Build history of the part. All positions in model axes, mm. A direction names the side the tool comes from. Round coordinates to 2 decimals unless told otherwise and drop trailing zeros. Write each loop counter-clockwise with the first axis right and the second up, starting at its lowest first coordinate (ties: lowest second). Pieces come first, ordered by that corner, then holes.
from build123d import *

# Parameters (mm, degrees)
ESQUISSE3_R             = 3
ENL_V_MAT_EXTRU_1_DEPTH = 11


with BuildPart() as part:
    # Esquisse1 → Révolution1 (revolve)
    with BuildSketch(Plane.XY, mode=Mode.PRIVATE) as r_volution1_sk:
        Polygon((0, 0), (30, 0), (30, 10), (7.4, 10), (7.4, 20), (0, 20), align=None)
    revolve(r_volution1_sk.sketch.rotate(Axis((0, 30.251396648, 0), (0, -1, 0)), 90), axis=Axis((0, 30.251396648, 0), (0, -1, 0)))  # turned: the seam where the file's is

    # Esquisse3 → Enlèv. mat.-Extru.1 (cut, through all)
    with BuildSketch(Plane(origin=(0, 10, 0), x_dir=(1, 0, 0), z_dir=(0, 1, 0))):
        with Locations(Location((0, 23, 0), (0, 0, 270))):  # turned: the seam where the file's is
            Circle(ESQUISSE3_R)
        with Locations(Location((19.918584287, -11.5, 0), (0, 0, 270))):  # turned: the seam where the file's is
            Circle(ESQUISSE3_R)
        with Locations(Location((-19.918584287, -11.5, 0), (0, 0, 270))):  # turned: the seam where the file's is
            Circle(ESQUISSE3_R)
    extrude(amount=-ENL_V_MAT_EXTRU_1_DEPTH, mode=Mode.SUBTRACT)


solid = part.part
1) Slice it at A-A (x = 0). Write the cut outline in (y, z).
Results:
outline: (0, -30) - (10, -30) - (10, -26) - (0, -26) - close; (0, -20) - (10, -20) - (10, -7.4) - (20, -7.4) - (20, 7.4) - (10, 7.4) - (10, 30) - (0, 30) - close
2) Slice it at B-B (z = 0). Write the cut outline in (x, y), plus the area to 3 significant figures.
Results:
outline: (-30, 0) - (30, 0) - (30, 10) - (7.4, 10) - (7.4, 20) - (-7.4, 20) - (-7.4, 10) - (-30, 10) - close
area: 748 mm2
3) Slice it at C-C (z = -23). Write the cut outline in (x, y).
Results:
outline: (-19.26, 0) - (-3, 0) - (-3, 10) - (-19.26, 10) - close; (3, 0) - (19.26, 0) - (19.26, 10) - (3, 10) - close
4) Pin check, flat tips, straight feed: pin 1 Ø10 at (x, y) = (-14.5, 7) entering from -Z; pin 2 Ø3 at (y, z) = (7, 2.5) entering from +X; pin 3 Ø10 at (y, z) = (4.5, -20.5) entering from +X; pin 4 Ø6 at (x, z) = (0.5, 0) entering from -Y. Stop position of each tip, or through.
Results:
pin 1: stops at z = -28.46
pin 2: stops at x = 29.98
pin 3: stops at x = 25.69
pin 4: stops at y = 0
5) Which spindle directions (+Z, -Z, +X, -X, +Y, -Y) get a long thin tool onto all of the face, cutting with end or side? Do faces 4 (the cylindrical face through (21.95, 5.07, 9.29)), 5 (the cylindrical face through (7.224, 15.07, -1.604)). Say none if no direction does.
Results:
face 4: +Y, -Y
face 5: +Y
6) Wall check: L1, parallel to Y at x = 25.5, z = 1; L2, parallel to X at y = 18.5, z = 0; L3, parallel to X at y = 8.25, z = -23. Give the ranges that are in metal, low to high.
Results:
L1: y = 0 to 10
L2: x = -7.4 to 7.4
L3: x = -19.26 to -3, 3 to 19.26
7) Slice it at D-D (z = 11.5). Write the cut outline in (x, y).
Results:
outline: (-27.71, 0) - (-22.92, 0) - (-22.92, 10) - (-27.71, 10) - close; (-16.92, 0) - (16.92, 0) - (16.92, 10) - (-16.92, 10) - close; (22.92, 0) - (27.71, 0) - (27.71, 10) - (22.92, 10) - close
8) Mould opens along X. For faces 1 (the cylindrical face through (-25.296, 5.07, 16.128)), 2 (the flat face through (6, 10, 6)), 3 (the cylindrical face through (-16.944, 5.07, 11.109)) say: released by +X, released by -X, zero draft, split by the parting line, or undercut.
Results:
face 1: split by the parting line
face 2: zero draft
face 3: undercut
